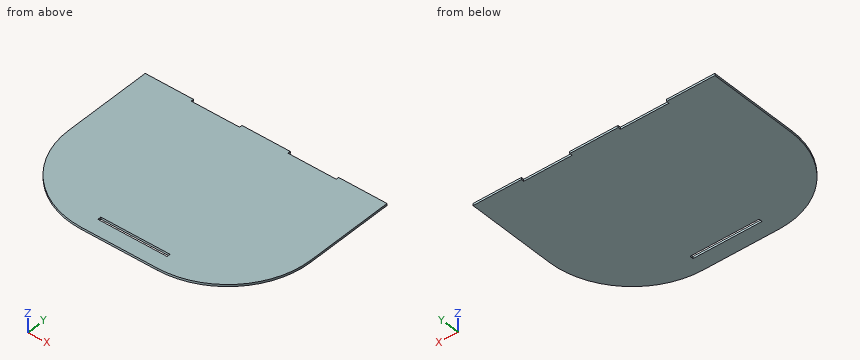
from build123d import *

# Parameters (mm, degrees)
F0_W     = 100
F0_H     = 5
F0_W_2   = 70
F0_H_2   = 4
F1_DEPTH = 3
F2_R     = 120


with BuildPart() as f1:
    # F0 (on Top) → F1 (new body)
    with BuildSketch(Plane.XY):
        Polygon((0, 246), (0, 0), (350, 0), (350, 246), (280, 246), (210, 246), (140, 246), (70, 246), align=None)
        with Locations((175, 25)):
            Rectangle(F0_W, F0_H, mode=Mode.SUBTRACT)
        with Locations((175, 248)):
            Rectangle(F0_W_2, F0_H_2)
        with Locations((315, 248)):
            Rectangle(F0_W_2, F0_H_2)
        with Locations((35, 248)):
            Rectangle(F0_W_2, F0_H_2)
    extrude(amount=F1_DEPTH)

    # F2
    f2_edges = [f1.edges().sort_by_distance(p)[0] for p in [
        (0, 0, 1.5),
        (350, 0, 1.5),
    ]]
    fillet(f2_edges, radius=F2_R)


solid = f1.part
The model under review builds one solid part; all positions refer to its coordinate system, in mm. Round coordinates to 2 decimals unless told otherwise and drop trailing zeros. Loops run counter-clockwise (first coordinate to the right, second up) from the corner with the lowest first, then second, coordinate; pieces in that order, holes last. Notation, with made-up numbers: (48, 68) - (66, 68) arc R28 cw to (66, 107) - close; hole circle Ø9 at (59.5, 52.25). An arc over 180 degrees is marked (long way). Use CSV: the item, a comma, the result in double quotes.
(1) For line 1 (Y direction, x = 178.5, z = 1.8); line 2 (Y direction, x = 134, z = 0.85); line 3 (X direction, y = 66, z = 2.95), list the stretches that pass through material, from the lowest coordinate up.
Working result:
line 1,"y = 0 to 22.5, 27.5 to 250"
line 2,"y = 0 to 22.5, 27.5 to 246"
line 3,"x = 12.84 to 337.16"
(2) Clearance check with a flat-ended pin moving along its axis: P1, Ø1.5, axis at x = 253.5, z = 1, coming from the +Y side. State where the tip first meets the part, or that it passes through.
Working result:
P1,"stops at y = 246"
(3) Take a section at A-A, the plane x = 173. Give the boundary of the cut face in (y, z).
Working result:
outline,"(0, 0) - (22.5, 0) - (22.5, 3) - (0, 3) - close; (27.5, 0) - (250, 0) - (250, 3) - (27.5, 3) - close"
(4) Take a section at C-C, the plane y = 72.5. Give the boundary of the cut face in (x, z), plus the area to 3 significant figures.
Working result:
outline,"(9.8, 0) - (340.2, 0) - (340.2, 3) - (9.8, 3) - close"
area,"991 mm^2"
(5) Take a section at D-D, the plane x = 57.5. Give the boundary of the cut face in (y, z).
Working result:
outline,"(17.56, 0) - (250, 0) - (250, 3) - (17.56, 3) - close"
(6) Take a section at B-B, the plane z = 2.5. Give the boundary of the cut face in (x, y).
Working result:
outline,"(0, 120) arc R120 ccw to (120, 0) - (230, 0) arc R120 ccw to (350, 120) - (350, 250) - (280, 250) - (280, 246) - (210, 246) - (210, 250) - (140, 250) - (140, 246) - (70, 246) - (70, 250) - (0, 250) - close; hole (125, 22.5) - (225, 22.5) - (225, 27.5) - (125, 27.5) - close"
